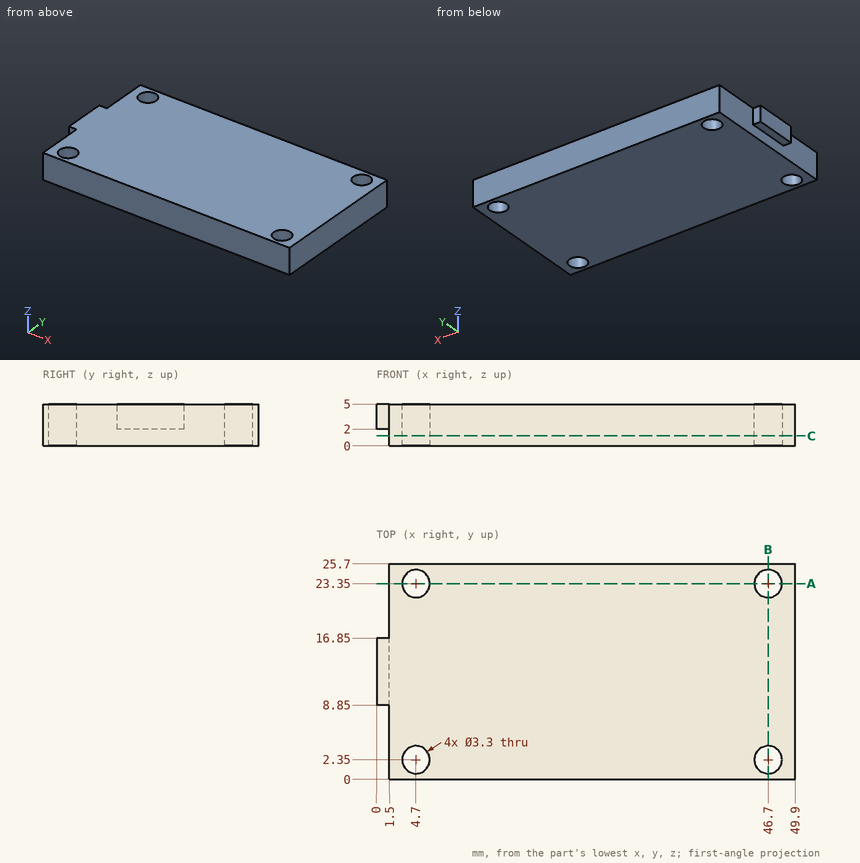
Answer from the drawing. Dimensions are ordinates in mm from the lowest x, y and z of the part. Give positions to 0.01 mm unless a question says otherwise; leave off trailing zeros. Order: outer loops, then holes, each group sorted by start corner. A loop starts at its lowest first (then second) coordinate and runs counter-clockwise, first axis right, second up. Notation, with made-up numbers: (-12, 62) - (12, 62) arc R20 cw to (12, 70) - close; hole circle Ø2 at (61.5, 33.25). An arc over 180 degrees is marked (long way). One line per item, written item: value. Start each with the question number.
1. Section A-A, the plane y = 23.35 is taken. Write down the section's boundary in (x, z).
2. Each of these flat-tipped pins is pushed along its axis until it touches: pin 1 Ø0.8 at (x, y) = (1, 14.5) entering from -Z; pin 2 Ø1.5 at (y, z) = (7, 3) entering from -X. Where does it stop, or does it pass through?
3. Section B-B, the plane x = 46.7 is taken. Write down the section's boundary in (y, z).
4. Consider line 1 (Y direction, x = 4.7, z = 3.9); line 2 (X direction, y = 23.75, z = 0.35); line 3 (X direction, y = 3.5, z = 3.45). Determine where each line is inside the solid, lowest interval first.
5. Section C-C, the plane z = 1.2 is taken. Write down the section's boundary in (x, y), then the cut area to 3 significant figures.
Filled sheet:
1. outline: (1.5, 0) - (3.05, 0) - (3.05, 5) - (1.5, 5) - close; (6.35, 0) - (45.05, 0) - (45.05, 5) - (6.35, 5) - close; (48.35, 0) - (49.9, 0) - (49.9, 5) - (48.35, 5) - close
2. pin 1: z = 2
2. pin 2: x = 1.5
3. outline: (0, 0) - (0.7, 0) - (0.7, 5) - (0, 5) - close; (4, 0) - (21.7, 0) - (21.7, 5) - (4, 5) - close; (25, 0) - (25.7, 0) - (25.7, 5) - (25, 5) - close
4. line 1: 0 to 0.7, 4 to 21.7, 25 to 25.7
4. line 2: 1.5 to 3.1, 6.3 to 45.1, 48.3 to 49.9
4. line 3: 1.5 to 3.52, 5.88 to 45.52, 47.88 to 49.9
5. outline: (1.5, 0) - (49.9, 0) - (49.9, 25.7) - (1.5, 25.7) - close; hole circle Ø3.3 at (4.7, 2.35); hole circle Ø3.3 at (4.7, 23.35); hole circle Ø3.3 at (46.7, 2.35); hole circle Ø3.3 at (46.7, 23.35)
5. area: 1,210 mm²
